```python
from build123d import *

# Parameters (mm, degrees)
CROQUIS1_W              = 50.8
CROQUIS1_H              = 50.8
CROQUIS1_W_2            = 44.8
CROQUIS1_H_2            = 44.8
SALIENTE_EXTRUIR1_DEPTH = 250
CROQUIS2_R              = 6.35
CORTAR_EXTRUIR1_DEPTH   = 257.370435113


with BuildPart() as part:
    # Croquis1 → Saliente-Extruir1 (new, symmetric)
    with BuildSketch(Plane.XY):
        Rectangle(CROQUIS1_W, CROQUIS1_H)
        Rectangle(CROQUIS1_W_2, CROQUIS1_H_2, mode=Mode.SUBTRACT)
    extrude(amount=SALIENTE_EXTRUIR1_DEPTH, both=True)

    # Croquis2 → Cortar-Extruir1 (cut, through all)
    with BuildSketch(Plane(origin=(25.4, 0, 0), x_dir=(0, 0, -1), z_dir=(1, 0, 0))):
        with Locations((-223, 0)):
            Circle(CROQUIS2_R)
        with Locations(Location((235, 0, 0), (0, 0, 270))):
            Circle(CROQUIS2_R)
    extrude(amount=-CORTAR_EXTRUIR1_DEPTH, mode=Mode.SUBTRACT)


solid = part.part
```
Here's how the part is built. I have some questions about the finished solid (model axes, mm). A direction names the side the tool comes from. Give positions to 0.01 mm unless a question says otherwise; leave off trailing zeros. Order: outer loops, then holes, each group sorted by start corner. A loop starts at its lowest first (then second) coordinate and runs counter-clockwise, first axis right, second up. Notation, with made-up numbers: (36.25, 50) -> (51.25, 50) arc R18 cw to (51.25, 69) -> close; hole circle Ø2 at (64.25, 86.25). An arc over 180 degrees is marked (long way). Use CSV: the item, a comma, the result in double quotes. Start each with the question number.
Item 1: Suppose I cut it at C-C (x = -15.5). List the corners of the cut face in (y, z) for me.
Item 2: Suppose I cut it at A-A (y = 0). List the corners of the cut face in (x, z) for me.
Item 3: On a 3-axis mill with a long thin cutter (end or side, diameter ignored), from which of +Z, -Z, +X, -X, +Y, -Y can I reach the whole of each face in a straight line? I mean faces 4 (the flat face through (-23, 0, -250)), 5 (the flat face through (0, 22.4, 4)). Say none if no direction works.
Item 4: Thinking about a two-plate mould opening in Z: for faces 1 (the cylindrical face through (23.921, 1.907, 216.943)), 2 (the flat face through (-23, 0, 250)), 3 (the flat face through (0, -22.4, 4)), which applies, pulls with the +Z half, pulls with the -Z half, needs draft (parallel to the pull), parting line crosses it, or undercut?
Item 5: Suppose I cut it at B-B (z = 223). List the corners of the cut face in (x, y) for me, and give its area (3 significant figures).
Item 6: If I drill on probe 1 along Y at (x, z) = (23.8, -235); probe 2 along X at (y, z) = (3, -63.5), over which ranges is the centre line in solid material (lowest first)? Write a range as [from, to].
Answer block:
1,outline,"(-25.4, -250) -> (-22.4, -250) -> (-22.4, 250) -> (-25.4, 250) -> close; (22.4, -250) -> (25.4, -250) -> (25.4, 250) -> (22.4, 250) -> close"
2,outline,"(-25.4, -250) -> (-22.4, -250) -> (-22.4, -241.35) -> (-25.4, -241.35) -> close; (-25.4, -228.65) -> (-22.4, -228.65) -> (-22.4, 216.65) -> (-25.4, 216.65) -> close; (-25.4, 229.35) -> (-22.4, 229.35) -> (-22.4, 250) -> (-25.4, 250) -> close; (22.4, -250) -> (25.4, -250) -> (25.4, -241.35) -> (22.4, -241.35) -> close; (22.4, -228.65) -> (25.4, -228.65) -> (25.4, 216.65) -> (22.4, 216.65) -> close; (22.4, 229.35) -> (25.4, 229.35) -> (25.4, 250) -> (22.4, 250) -> close"
3,face 4,"-Z, +X, -X, +Y, -Y"
3,face 5,"+Z, -Z"
4,face 1,"undercut"
4,face 2,"pulls with the +Z half"
4,face 3,"needs draft"
5,outline,"(-25.4, -25.4) -> (25.4, -25.4) -> (25.4, -6.35) -> (22.4, -6.35) -> (22.4, -22.4) -> (-22.4, -22.4) -> (-22.4, -6.35) -> (-25.4, -6.35) -> close; (-25.4, 6.35) -> (-22.4, 6.35) -> (-22.4, 22.4) -> (22.4, 22.4) -> (22.4, 6.35) -> (25.4, 6.35) -> (25.4, 25.4) -> (-25.4, 25.4) -> close"
5,area,"497 mm^2"
6,probe 1,"y = [-25.4, -6.35], [6.35, 25.4]"
6,probe 2,"x = [-25.4, -22.4], [22.4, 25.4]"
